The figure shows three views and two pictorial views of one solid part (mm, origin at its lowest corner). Answer the questions. A direction names the side the tool comes from. Coordinates: 2 decimals unless noted, no trailing zeros. Loops run counter-clockwise (first coordinate to the right, second up) from the corner with the lowest first, then second, coordinate; pieces in that order, holes last. Notation, with made-up numbers: (58, -14) - (113, -14) arc R17 cw to (113, 5) - close; hole circle Ø2 at (79, -27.75). An arc over 180 degrees is marked (long way). Return JSON: item names as keys, results as strings. Group by question number.
1. Find the intervals of material crossed by line 1 along X through (y, z) = (35.5, 5); line 2 along Y through (x, z) = (76.5, 5); line 3 along Y through (x, z) = (5, 2.75), in increasing order.
2. Which of the six approach directions +Z, -Z, +X, -X, +Y, -Y give full straight-line access (tool end or side, diameter ignored) to the marked faces 1 and 2?
3. The mould has two halves that part along X. Classify the marked faces 3 and 4: pulls with the +X half, pulls with the -X half, needs draft (parallel to the pull), parting line crosses it, or undercut.
4. Section B-B (x = 5) is taken. Write down the section's boundary in (y, z).
5. Section C-C (z = 2) is taken. Write down the section's boundary in (x, y).
6. Section A-A (y = 57.5) is taken. Write down the section's boundary in (x, z).
7. Each of these flat-tipped pins is pushed along its axis until it touches: P1, Ø2, axis at x = 114, z = 3, coming from the -Y side; P2, Ø6, axis at y = 2.5, z = 3, coming from the +X side; P3, Ø10, axis at x = 94, y = 70.5, coming from the -Z side. Where does it stop, or does it pass through?
8. Section D-D (y = 18) is taken. Write down the section's boundary in (x, z), and give its area (3 significant figures).
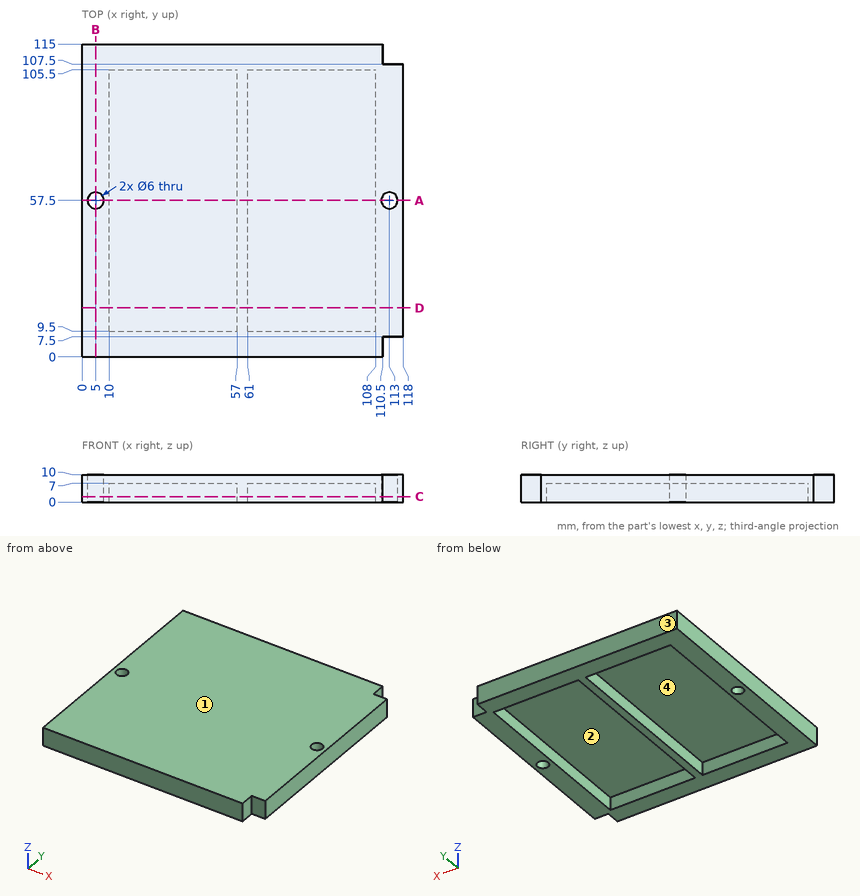
The answers:
{
 "1": {"line 1": "x = 0 to 10, 57 to 61, 108 to 118", "line 2": "y = 0 to 9.5, 105.5 to 115", "line 3": "y = 0 to 54.5, 60.5 to 115"},
 "2": {"face 1": "+Z, +X, -X, +Y, -Y", "face 2": "-Z"},
 "3": {"face 3": "needs draft", "face 4": "undercut"},
 "4": {"outline": "(0, 0) - (54.5, 0) - (54.5, 10) - (0, 10) - close; (60.5, 0) - (115, 0) - (115, 10) - (60.5, 10) - close"},
 "5": {"outline": "(0, 0) - (110.5, 0) - (110.5, 7.5) - (118, 7.5) - (118, 107.5) - (110.5, 107.5) - (110.5, 115) - (0, 115) - close; hole circle Ø6 at (5, 57.5); hole (10, 9.5) - (57, 9.5) - (57, 105.5) - (10, 105.5) - close; hole (61, 9.5) - (108, 9.5) - (108, 105.5) - (61, 105.5) - close; hole circle Ø6 at (113, 57.5)"},
 "6": {"outline": "(0, 0) - (2, 0) - (2, 10) - (0, 10) - close; (8, 0) - (10, 0) - (10, 7) - (57, 7) - (57, 0) - (61, 0) - (61, 7) - (108, 7) - (108, 0) - (110, 0) - (110, 10) - (8, 10) - close; (116, 0) - (118, 0) - (118, 10) - (116, 10) - close"},
 "7": {"P1": "stops at y = 7.5", "P2": "stops at x = 110.5", "P3": "stops at z = 7"},
 "8": {"outline": "(0, 0) - (10, 0) - (10, 7) - (57, 7) - (57, 0) - (61, 0) - (61, 7) - (108, 7) - (108, 0) - (118, 0) - (118, 10) - (0, 10) - close", "area": "522 mm2"}
}
